Part model, mm, in its own coordinate system. Round coordinates to 2 decimals unless told otherwise and drop trailing zeros. Order: outer loops, then holes, each group sorted by start corner. A loop starts at its lowest first (then second) coordinate and runs counter-clockwise, first axis right, second up. Notation, with made-up numbers: (20, 47) -> (47, 47) arc R11 cw to (47, 63) -> close; hole circle Ø3 at (12.25, -12). An arc over 180 degrees is marked (long way). Return JSON: item names as keys, results as strings. Group by question number.
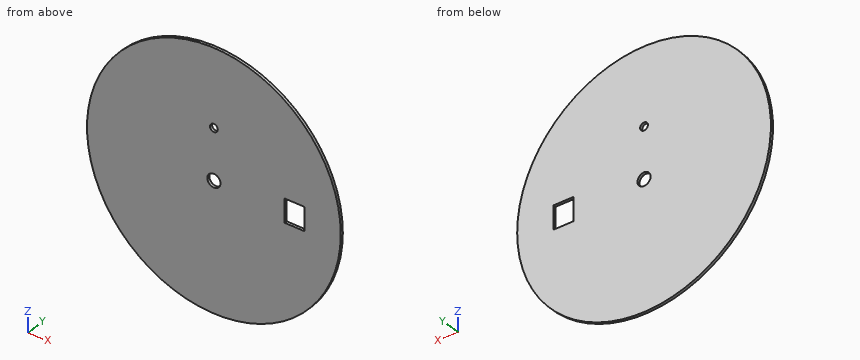
Autodesk Fusion 360 part; units mm, degrees
sketch "Sketch1" plane through (0, 0, 0) normal (0, 1, 0) x (1, 0, 0)
  circle A0 centre (0, 0) radius 16.375
  dimension "d1" = 32.75
extrude "Extrude1" add sketch "Sketch1" along normal blind 0.35
sketch "Sketch3" plane through (0, 0.35, 0) normal (0, 1, 0) x (-1, 0, 0)
  circle A0 centre (0, 0) radius 16.375
  circle A1 centre (0, 0) radius 0.85
  line L0 (-9.1, 1.5) -> (-11.7, 1.5)
  line L1 (-11.7, 1.5) -> (-11.7, -1.5)
  line L2 (-11.7, -1.5) -> (-9.1, -1.5)
  line L3 (-9.1, -1.5) -> (-9.1, 1.5)
  circle A2 centre (0, 6.5) radius 0.5
  dimension "d4" = 1.7
  dimension "d5" = 2.6
  dimension "d6" = 3
  dimension "d7" = 1.5
  dimension "d8" = 9.1
  dimension "d9" = 1
  dimension "d10" = 6.5
extrude "Extrude2" cut sketch "Sketch3" against normal through all contours A1 | L0 L1 L2 L3 | A2
sketch "Sketch4" plane through (0, 0.35, 0) normal (0, 1, 0) x (-1, 0, 0)
  line L0 (-9.1, -1.5) -> (-11.7, -1.5)
  line L1 (-11.7, -1.5) -> (-11.7, 1.5)
  line L2 (-11.7, 1.5) -> (-9.1, 1.5)
  line L3 (-9.1, 1.5) -> (-9.1, -1.5)
  circle A0 centre (0, 0) radius 0.85
  circle A1 centre (0, 6.5) radius 0.5
  circle A2 centre (0, 0) radius 16.375
  line L4 (0.375, 12.5) -> (-0.375, 12.5)
  line L5 (-0.375, 12.5) -> (-0.375, 14.5)
  line L6 (-0.375, 14.5) -> (0.375, 14.5)
  line L7 (0.375, 14.5) -> (0.375, 12.5)
  line L8 (-6.5748, 10.6378) -> (-7.5748, 12.3699)
  line L9 (-6.9252, 12.7449) -> (-5.9252, 11.0128)
  line L10 (-5.9252, 11.0128) -> (-6.5748, 10.6378)
  line L11 (-7.5748, 12.3699) -> (-6.9252, 12.7449)
  line L12 (-11.0128, 5.9252) -> (-12.7449, 6.9252)
  line L13 (-12.3699, 7.5748) -> (-10.6378, 6.5748)
  line L14 (-10.6378, 6.5748) -> (-11.0128, 5.9252)
  line L15 (-12.7449, 6.9252) -> (-12.3699, 7.5748)
  line L16 (-12.5, -0.375) -> (-14.5, -0.375)
  line L17 (-14.5, 0.375) -> (-12.5, 0.375)
  line L18 (-12.5, 0.375) -> (-12.5, -0.375)
  line L19 (-14.5, -0.375) -> (-14.5, 0.375)
  line L20 (-10.6378, -6.5748) -> (-12.3699, -7.5748)
  line L21 (-12.7449, -6.9252) -> (-11.0128, -5.9252)
  line L22 (-11.0128, -5.9252) -> (-10.6378, -6.5748)
  line L23 (-12.3699, -7.5748) -> (-12.7449, -6.9252)
  line L24 (-5.9252, -11.0128) -> (-6.9252, -12.7449)
  line L25 (-7.5748, -12.3699) -> (-6.5748, -10.6378)
  line L26 (-6.5748, -10.6378) -> (-5.9252, -11.0128)
  line L27 (-6.9252, -12.7449) -> (-7.5748, -12.3699)
  line L28 (6.5748, -10.6378) -> (7.5748, -12.3699)
  line L29 (6.9252, -12.7449) -> (5.9252, -11.0128)
  line L30 (5.9252, -11.0128) -> (6.5748, -10.6378)
  line L31 (7.5748, -12.3699) -> (6.9252, -12.7449)
  line L32 (11.0128, -5.9252) -> (12.7449, -6.9252)
  line L33 (12.3699, -7.5748) -> (10.6378, -6.5748)
  line L34 (10.6378, -6.5748) -> (11.0128, -5.9252)
  line L35 (12.7449, -6.9252) -> (12.3699, -7.5748)
  line L36 (12.5, 0.375) -> (14.5, 0.375)
  line L37 (14.5, -0.375) -> (12.5, -0.375)
  line L38 (12.5, -0.375) -> (12.5, 0.375)
  line L39 (14.5, 0.375) -> (14.5, -0.375)
  line L40 (10.6378, 6.5748) -> (12.3699, 7.5748)
  line L41 (12.7449, 6.9252) -> (11.0128, 5.9252)
  line L42 (11.0128, 5.9252) -> (10.6378, 6.5748)
  line L43 (12.3699, 7.5748) -> (12.7449, 6.9252)
  line L44 (5.9252, 11.0128) -> (6.9252, 12.7449)
  line L45 (7.5748, 12.3699) -> (6.5748, 10.6378)
  line L46 (6.5748, 10.6378) -> (5.9252, 11.0128)
  line L47 (6.9252, 12.7449) -> (7.5748, 12.3699)
  line L48 (0.75, -14.5) -> (-0.75, -14.5)
  line L49 (-0.75, -14.5) -> (0, -11.75)
  line L50 (0, -11.75) -> (0.75, -14.5)
  line L51 (0, -14.5) -> (0, -11.75)
  line L52 (-5, 6.5) -> (-4, 6.5)
  line L53 (-4.3301, 4) -> (-3.4641, 4.5)
  line L54 (-2.5, 2.1699) -> (-2, 3.0359)
  line L55 (0, 1.5) -> (0, 2.5)
  line L56 (2.5, 2.1699) -> (2, 3.0359)
  line L57 (4.3301, 4) -> (3.4641, 4.5)
  line L58 (5, 6.5) -> (4, 6.5)
  line L59 (4.3301, 9) -> (3.4641, 8.5)
  line L60 (2.5, 10.8301) -> (2, 9.9641)
  line L61 (0, 11.5) -> (0, 10.5)
  line L62 (-2.5, 10.8301) -> (-2, 9.9641)
  line L63 (-4.3301, 9) -> (-3.4641, 8.5)
  dimension "d12" = 0.75
  dimension "d13" = 2
  dimension "d14" = 14.5
  dimension "d15" = 0.375
  dimension "d17" = 360
  dimension "d18" = 2.75
  dimension "d19" = 1.5
  dimension "d20" = 14.5
  dimension "d21" = 0.75
  dimension "d24" = 5
  dimension "d25" = 1
  dimension "d27" = 360
sketch "Sketch5" plane through (0, 0.35, 0) normal (0, 1, 0) x (-1, 0, 0)
  line L0 (6.985, -3.5778) -> (-7.6268, -3.5778) construction
  line L1 (-7.6268, -3.5778) -> (-7.6268, -6.5778) construction
  line L2 (-7.6268, -6.5778) -> (6.985, -6.5778) construction
  line L3 (6.985, -6.5778) -> (6.985, -3.5778) construction
  line L4 (0.4767, -9.049) -> (-0.7965, -9.049) construction
  line L5 (-0.7965, -9.049) -> (-0.7965, -11.549) construction
  line L6 (-0.7965, -11.549) -> (0.4767, -11.549) construction
  line L7 (0.4767, -11.549) -> (0.4767, -9.049) construction
  line L8 (-5.4546, -8.2) -> (-5.7, -8.2) construction
  line L9 (-5.7, -8.2) -> (-5.7, -10.7) construction
  line L10 (-5.7, -10.7) -> (-5.4546, -10.7) construction
  line L11 (-5.4546, -10.7) -> (-5.4546, -8.2) construction
  line L12 (-9.0419, -4.874) -> (-9.8, -4.874) construction
  line L13 (-9.8, -4.874) -> (-9.8, -7.374) construction
  line L14 (-9.8, -7.374) -> (-9.0419, -7.374) construction
  line L15 (-9.0419, -7.374) -> (-9.0419, -4.874) construction
  line L16 (-9.1553, 6.5) -> (-10, 6.5) construction
  line L17 (-10, 6.5) -> (-10, 4) construction
  line L18 (-10, 4) -> (-9.1553, 4) construction
  line L19 (-9.1553, 4) -> (-9.1553, 6.5) construction
  line L20 (-5.2603, 10) -> (-6, 10) construction
  line L21 (-6, 10) -> (-6, 7.5) construction
  line L22 (-6, 7.5) -> (-5.2603, 7.5) construction
  line L23 (-5.2603, 7.5) -> (-5.2603, 10) construction
  line L24 (5.6618, -8.1907) -> (4.9086, -8.1907) construction
  line L25 (4.9086, -8.1907) -> (4.9086, -10.6907) construction
  line L26 (4.9086, -10.6907) -> (5.6618, -10.6907) construction
  line L27 (5.6618, -10.6907) -> (5.6618, -8.1907) construction
  line L28 (5.7568, 10.0139) -> (5, 10.0139) construction
  line L29 (5, 10.0139) -> (5, 7.5139) construction
  line L30 (5, 7.5139) -> (5.7568, 7.5139) construction
  line L31 (5.7568, 7.5139) -> (5.7568, 10.0139) construction
  line L32 (9.7568, 6.5) -> (8.9817, 6.5) construction
  line L33 (8.9817, 6.5) -> (8.9817, 4) construction
  line L34 (8.9817, 4) -> (9.7568, 4) construction
  line L35 (9.7568, 4) -> (9.7568, 6.5) construction
  line L36 (11.2571, 0.9949) -> (10.5002, 0.9949) construction
  line L37 (10.5002, 0.9949) -> (10.5002, -1.5051) construction
  line L38 (10.5002, -1.5051) -> (11.2571, -1.5051) construction
  line L39 (11.2571, -1.5051) -> (11.2571, 0.9949) construction
  line L40 (9.7568, -4.9) -> (8.4141, -4.9) construction
  line L41 (8.4141, -4.9) -> (8.4141, -7.4) construction
  line L42 (8.4141, -7.4) -> (9.7568, -7.4) construction
  line L43 (9.7568, -7.4) -> (9.7568, -4.9) construction
(1) Probe L1, parallel to Z at x = 0, y = 0.1 (3 decimals); L2, parallel to X at y = 0.1, z = 8; L3, parallel to X at y = 0.25, z = -2. List the from-to ranges inside material, lowest first. Write a range as [from, to].
(2) Pin check, flat tip, straight feed: P1, Ø1.5, axis at x = 0, z = 0, coming from the +Y side. Stop position of the tip, or through.
(3) Saw through at C-C, the plane y = 0.1. List the corners of the cut face in (x, z) (3 decimals), and give its area (3 significant figures).
(4) Saw through at D-D, the plane z = 6.5. List the corners of the cut face in (x, y), and give its area (3 significant figures).
(5) Saw through at B-B, the plane z = 0. List the corners of the cut face in (x, y) (3 decimals), and give its area (3 significant figures).
(6) Saw through at A-A, the plane x = 0. List the corners of the cut face in (y, z) (3 decimals), and give its area (3 significant figures).
Results are:
{
 "1": {"L1": "z = [-16.375, -0.85], [0.85, 6], [7, 16.375]", "L2": "x = [-14.29, 14.29]", "L3": "x = [-16.25, 16.25]"},
 "2": {"P1": "passes through"},
 "3": {"outline": "circle Ø32.75 at (0, 0); hole circle Ø1.7 at (0, 0); hole circle Ø1 at (0, 6.5); hole (9.1, -1.5) -> (11.7, -1.5) -> (11.7, 1.5) -> (9.1, 1.5) -> close", "area": "832 mm^2"},
 "4": {"outline": "(-15.03, 0) -> (-0.5, 0) -> (-0.5, 0.35) -> (-15.03, 0.35) -> close; (0.5, 0) -> (15.03, 0) -> (15.03, 0.35) -> (0.5, 0.35) -> close", "area": "10.2 mm^2"},
 "5": {"outline": "(-16.375, 0) -> (-0.85, 0) -> (-0.85, 0.35) -> (-16.375, 0.35) -> close; (0.85, 0) -> (9.1, 0) -> (9.1, 0.35) -> (0.85, 0.35) -> close; (11.7, 0) -> (16.375, 0) -> (16.375, 0.35) -> (11.7, 0.35) -> close", "area": "9.96 mm^2"},
 "6": {"outline": "(0, -16.375) -> (0.35, -16.375) -> (0.35, -0.85) -> (0, -0.85) -> close; (0, 0.85) -> (0.35, 0.85) -> (0.35, 6) -> (0, 6) -> close; (0, 7) -> (0.35, 7) -> (0.35, 16.375) -> (0, 16.375) -> close", "area": "10.5 mm^2"}
}
